For this review, take the finished solid that the model builds, in its own axes (mm). Face numbers are marked on the shaded views. A direction names the side the tool comes from. Coordinates: 2 decimals unless noted, no trailing zeros. Loops run counter-clockwise (first coordinate to the right, second up) from the corner with the lowest first, then second, coordinate; pieces in that order, holes last.
1. Take a section at A-A, the plane x = 0. State the section outline as (y, z) points, then the cut area to 3 significant figures.
2. Mouldability with a two-part tool opening along Y and no side actions: class the marked faces 1, 2, 3 and 4 as pulls with the +Y half, pulls with the -Y half, needs draft (parallel to the pull), parting line crosses it, or undercut.
3. Take a section at B-B, the plane z = 11.5. State the section outline as (x, y) points.
4. Take a section at D-D, the plane x = -13.5. State the section outline as (y, z) points.
5. Machinability: for the marked faces 5 and 6, which of the approach directions +Z, -Z, +X, -X, +Y, -Y give a long, thin tool a straight path to every point of the face, cutting with its end or side? Answer none if there is none.
6. Take a section at C-C, the plane y = 10.5. State the section outline as (x, z) points.
7. To check wall thickness, follow probe 1 along Y at (x, z) = (13.5, 0.9); probe 2 along X at (y, z) = (11.5, 1); probe 3 along Z at (x, y) = (-2.5, 17). State the ranges of each line that lie inside material, in increasing order.
8. Clearance check with flat-ended pins moving along their axes: P1, Ø5, axis at x = -5.5, y = 14.5, coming from the +Z side; P2, Ø3, axis at x = -13.5, z = 10.5, coming from the +Y side. State where each tip first meets the part, or that it passes through.
```python
from build123d import *

# Parameters (mm, degrees)
BOSS_EXTRUDE3_DEPTH = 21.5
SKETCH4_W           = 37
SKETCH4_H           = 12
CUT_EXTRUDE1_DEPTH  = 17
SKETCH5_R           = 2.1
CUT_EXTRUDE2_DEPTH  = 32.721443851
SKETCH6_R           = 1.7
CUT_EXTRUDE3_DEPTH  = 32.2449996


with BuildPart() as part:
    # Sketch3 → Boss-Extrude3 (new, symmetric)
    with BuildSketch(Plane(origin=(0, 0, 0), x_dir=(0, 0, -1), z_dir=(1, 0, 0))):
        Polygon((0, 0), (0, 20), (-3.90885, 20), (-15, 3.55669), (-15, 0), align=None)
    extrude(amount=BOSS_EXTRUDE3_DEPTH, both=True)

    # Sketch4 → Cut-Extrude1 (cut)
    with BuildSketch(Plane(origin=(0, 20, 0), x_dir=(1, 0, 0), z_dir=(0, 1, 0))):
        with Locations((0, -9)):
            Rectangle(SKETCH4_W, SKETCH4_H)
    extrude(amount=-CUT_EXTRUDE1_DEPTH, mode=Mode.SUBTRACT)

    # Sketch5 → Cut-Extrude2 (cut, through all)
    with BuildSketch(Plane.XY.offset(3)):
        with Locations((-13.5, 10)):
            Circle(SKETCH5_R)
        with Locations((13.5, 10)):
            Circle(SKETCH5_R)
    extrude(amount=-CUT_EXTRUDE2_DEPTH, mode=Mode.SUBTRACT)

    # Sketch6 → Cut-Extrude3 (cut, through all)
    with BuildSketch(Plane(origin=(0, 3, 0), x_dir=(1, 0, 0), z_dir=(0, 1, 0))):
        with Locations(Location((0, -10.5, 0), (0, 0, 270))):
            Circle(SKETCH6_R)
    extrude(amount=-CUT_EXTRUDE3_DEPTH, mode=Mode.SUBTRACT)


solid = part.part
```
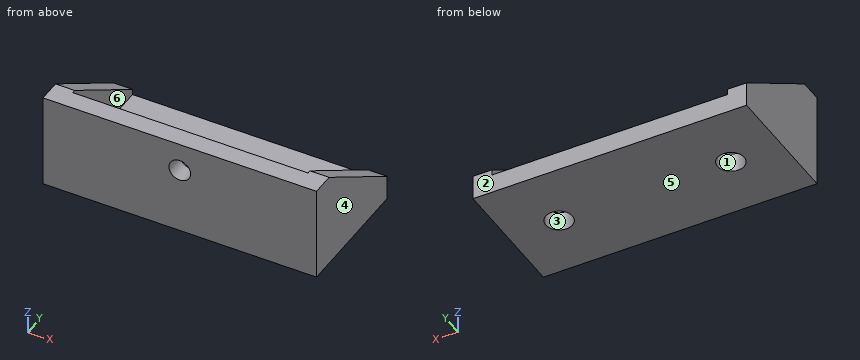
Results list:
1. outline: (0, 0) - (20, 0) - (20, 3) - (3, 3) - (3, 8.8) - (0, 8.8) - close; (0, 12.2) - (3, 12.2) - (3, 15) - (0, 15) - close
1. area: 85.8 mm2
2. face 1: undercut
2. face 2: pulls with the +Y half
2. face 3: undercut
2. face 4: needs draft
3. outline: (-21.5, 0) - (-1.37, 0) - (-1.37, 3) - (-18.5, 3) - (-18.5, 8.75) - (-21.5, 8.75) - close; (1.37, 0) - (21.5, 0) - (21.5, 8.75) - (18.5, 8.75) - (18.5, 3) - (1.37, 3) - close
4. outline: (0, 0) - (7.9, 0) - (7.9, 3) - (3, 3) - (3, 15) - (0, 15) - close; (12.1, 0) - (20, 0) - (20, 3) - (12.1, 3) - close
5. face 5: -Z, +X, -X, +Y, -Y
5. face 6: +Z, +Y
6. outline: (-21.5, 0) - (-15.54, 0) - (-15.54, 3) - (-18.5, 3) - (-18.5, 10.32) - (-21.5, 10.32) - close; (-11.46, 0) - (11.46, 0) - (11.46, 3) - (-11.46, 3) - close; (15.54, 0) - (21.5, 0) - (21.5, 10.32) - (18.5, 10.32) - (18.5, 3) - (15.54, 3) - close
7. probe 1: y = 0 to 7.9, 12.1 to 20
7. probe 2: x = -21.5 to -14.97, -12.03 to 12.03, 14.97 to 21.5
7. probe 3: z = 0 to 3
8. P1: stops at z = 3
8. P2: stops at y = 3
